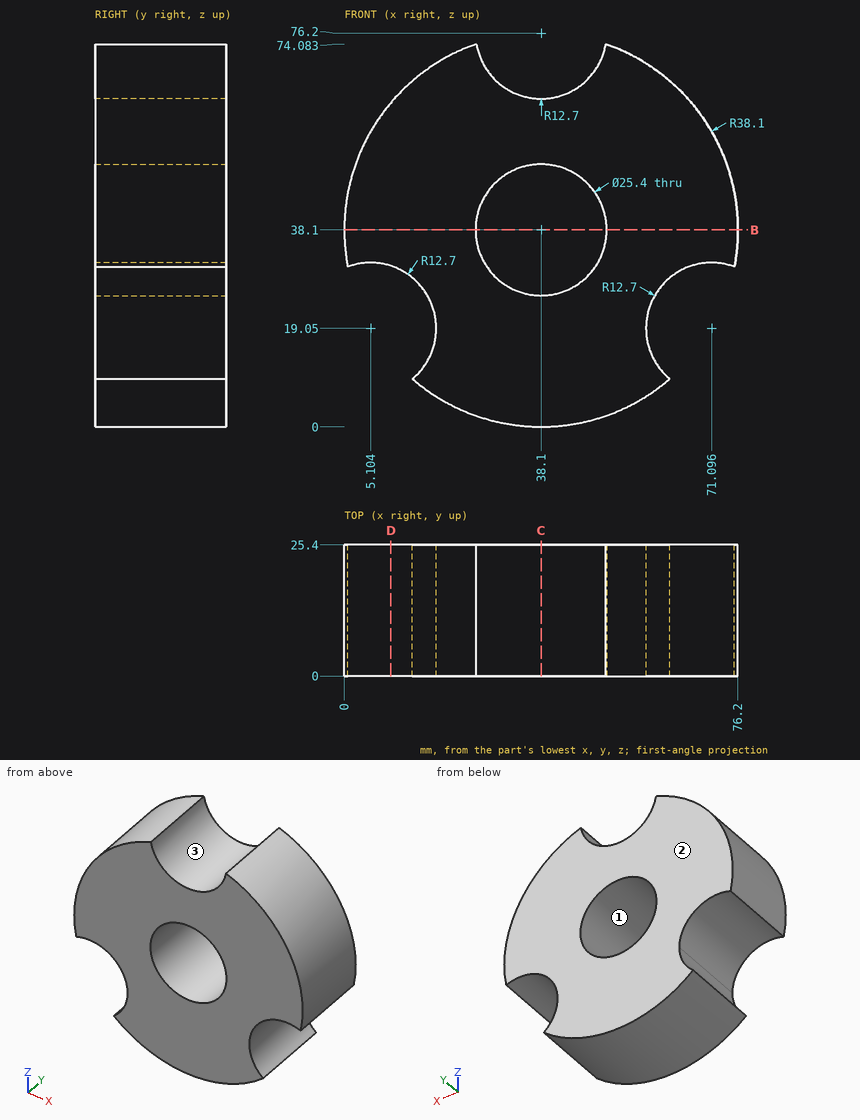
Input: dimensioned drawing with shaded views. Units: mm. Origin: part minimum x, y, z. Give positions to 0.01 mm unless a question says otherwise; leave off trailing zeros. Loops run counter-clockwise (first coordinate to the right, second up) from the corner with the lowest first, then second, coordinate; pieces in that order, holes last. Notation, with made-up numbers: (71.25, -10) - (107.25, -10) arc R23 ccw to (107.25, 15) - close; hole circle Ø5 at (64, 46). An arc over 180 degrees is marked (long way). Answer as CSV lines item,"result". Start each with the question number.
(1) Pin query (flat end, axial travel): P1, Ø8, axis at x = 66.5, y = 21.5, coming from the -Z side; P2, Ø6, axis at x = 13, y = 18, coming from the -Z side (1 decimal); P3, Ø6, axis at y = 7, z = 53.5, coming from the +X side (1 decimal). Return the tip coordinate at first contact, or that it passes through.
(2) Section query B-B (z = 38.1). Output: boundary loops of the cut face in (x, y), and give its area (3 significant figures).
(3) Section query C-C (x = 38.1). Output: boundary loops of the cut face in (y, z), and give its area (3 significant figures).
(4) Ray query, line 1 along Z through (x, y) = (38.5, 3); line 2 along X through (y, z) = (20.5, 28) (1 decimal); line 3 along Z through (x, y) = (16, 15.75) (1 decimal). Return the intervals inside material, ascending. Write a range as [from, to].
(5) Mould query, pull axis Z, two halves, no side actions, for the marked faces 1, 2 and 3. Classes: +Z half, -Z half, draft (parallel to the pull), parting line (faces both ways), or undercut.
(6) Section query D-D (x = 9). Output: boundary loops of the cut face in (y, z).
Worked answers:
1,P1,"stops at z = 8.84"
1,P2,"stops at z = 7.1"
1,P3,"stops at x = 74.1"
2,outline,"(0, 0) - (25.4, 0) - (25.4, 25.4) - (0, 25.4) - close; (50.8, 0) - (76.2, 0) - (76.2, 25.4) - (50.8, 25.4) - close"
2,area,"1,290 mm^2"
3,outline,"(0, 0) - (25.4, 0) - (25.4, 25.4) - (0, 25.4) - close; (0, 50.8) - (25.4, 50.8) - (25.4, 63.5) - (0, 63.5) - close"
3,area,"968 mm^2"
4,line 1,"z = [0, 25.41], [50.79, 63.51]"
4,line 2,"x = [14.1, 30.4], [45.8, 62.1]"
4,line 3,"z = [7.1, 12.5], [25.6, 69.1]"
5,face 1,"undercut"
5,face 2,"draft"
5,face 3,"+Z half"
6,outline,"(0, 31.14) - (25.4, 31.14) - (25.4, 62.69) - (0, 62.69) - close"
